from build123d import *

# Parameters (mm, degrees)
BOSS_EXTRUDE1_DEPTH         = 4.7625
F_3_4_0_75_DIAMETER_HOLE1_D = 19.05
F_6_CLEARANCE_HOLE1_D       = 4.3053


with BuildPart() as part:
    # Sketch1 → Boss-Extrude1 (new body)
    with BuildSketch(Plane.XY):
        with BuildLine():
            Line((-13.97, 22.86), (-13.97, 60.431603094))
            ThreePointArc((-13.97, 60.431603094), (-15.471871133, 62.5475), (-16.002, 65.0875))
            Line((-16.002, 65.0875), (-16.002, 81.28))
            Line((-16.002, 81.28), (-69.215, 57.912))
            Line((-69.215, 57.912), (-69.215, 22.86))
            Line((-69.215, 22.86), (-13.97, 22.86))
        make_face()
    extrude(amount=BOSS_EXTRUDE1_DEPTH)

    # 3/4 (0.75) Diameter Hole1 (through all)
    with Locations(Plane.XY.offset(4.7625)):
        with Locations((-41.275, 46.99)):
            Hole(F_3_4_0_75_DIAMETER_HOLE1_D / 2)

    # #6 Clearance Hole1 (through all)
    with Locations(Plane.XY.offset(4.7625)):
        with Locations((-56.896, 30.48), (-28.194, 68.072)):
            Hole(F_6_CLEARANCE_HOLE1_D / 2)


solid = part.part
Here's how the part is built. I have some questions about the finished solid (model axes, mm). A direction names the side the tool comes from. Round coordinates to 2 decimals unless told otherwise and drop trailing zeros. Loops run counter-clockwise (first coordinate to the right, second up) from the corner with the lowest first, then second, coordinate; pieces in that order, holes last.
1. For P1, Ø1.5, axis at x = -27.5, z = 2.5, coming from the +Y side; P2, Ø2.5, axis at y = 71, z = 1.5, coming from the +X side; P3, Ø1, axis at x = -30.5, z = 2.5, coming from the +Y side, each with a flat end and sliding along its axis, tell me the tip position at first contact or that it passes through.
Answer list:
P1: stops at y = 76.56
P2: stops at x = -16
P3: stops at y = 75.13
2. We'd pull the mould along X, two halves only. Please class faces 3 (the face through (-13.97, 41, 2)), 4 (the face through (-42.24, 69.76, 2.35)), 5 (the face through (-40.035, 56.434, 2.348)): +X half, -X half, draft (parallel to the pull), parting line (faces both ways), or undercut.
Answer list:
face 3: +X half
face 4: -X half
face 5: undercut
3. If I drill on line 1 along Y through (x, z) = (-55, 3.05); line 2 along X through (y, z) = (41, 3.55) (3 decimals); line 3 along Y through (x, z) = (-40, 3.9), over which ranges is the centre line in solid material (lowest first)?
Answer list:
line 1: y = 22.86 to 29.46, 31.5 to 64.15
line 2: x = -69.215 to -48.681, -33.869 to -13.97
line 3: y = 22.86 to 37.55, 56.43 to 70.74
4. If we section it at C-C on z = 2.35: Count the separate pieces of the cut face and the enclosed holes in it, plus the area to 3 significant figures.
Answer list:
separate pieces: 1
enclosed holes: 3
area: 2,250 mm2
5. Which directions (+Z, -Z, +X, -X, +Y, -Y) give clear straight access to the entire face, cutting with the end or side of a thin tool? Please do faces 1 (the face through (-30, 46, 0)), 2 (the face through (-16.002, 73, 2)).
Answer list:
face 1: -Z, +X, -X, +Y, -Y
face 2: +Z, -Z, +X, +Y
6. If we section it at B-B on x = -41.5: Write out the boundary of the cut face in (y, z).
Answer list:
outline: (22.86, 0) - (37.47, 0) - (37.47, 4.76) - (22.86, 4.76) - close; (56.51, 0) - (70.08, 0) - (70.08, 4.76) - (56.51, 4.76) - close
